Read the model definition and answer for the solid it produces. Units are mm, in the model's axes. Face numbers are marked on the shaded views. A direction names the side the tool comes from. Round coordinates to 2 decimals unless told otherwise and drop trailing zeros. Write each loop counter-clockwise with the first axis right and the second up, starting at its lowest first coordinate (ties: lowest second). Pieces come first, ordered by that corner, then holes. Notation, with made-up numbers: (17, -10) - (49, -10) arc R22 cw to (49, 18) - close; hole circle Ø7 at (70.5, 37.5). An arc over 180 degrees is marked (long way). Answer as CSV lines item,"result". Start each with the question number.
1) Find section B-B on x = -5.5. Determine the outline of the cut face in (y, z).
2) Consider line 1 along Y through (x, z) = (-105, 4.3); line 2 along Y through (x, z) = (-10, -4.5); line 3 along Y through (x, z) = (-31, 0.25). Determine where each line is inside the solid, lowest interval first.
3) For a pull along Y with two mould halves and no side action, classify the marked faces 4, 5, 6 and 7 as +Y half, -Y half, draft (parallel to the pull), parting line (faces both ways), or undercut.
4) Which of the six approach directions +Z, -Z, +X, -X, +Y, -Y give full straight-line access (tool end or side, diameter ignored) to the marked faces 1, 2 and 3?
5) Find section C-C on x = -31. Determine the outline of the cut face in (y, z), then the cut area to 3 significant figures.
6) Find section A-A on x = 10. Determine the outline of the cut face in (y, z).
7) Each of these flat-tipped pins is pushed along its axis until it touches: pin 1 (1.1 mm diameter, centred on y = 9, z = -4, fed in from +X); pin 2 (1.5 mm diameter, centred on y = 1, z = -3, fed in from +X); pin 3 (6 mm diameter, centred on x = 5.5, y = 1, fed in from -Z); pin 4 (3 mm diameter, centred on x = -105, y = -10, fed in from -Z). Where does it stop, or does it pass through?
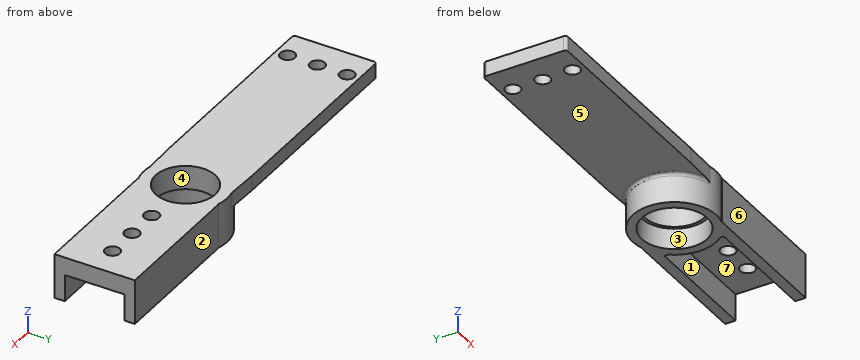
from build123d import *

# Parameters (mm, degrees)
SKETCH_1_W          = 40
SKETCH_1_H          = 20
EXTRUDE_1_DEPTH     = 6
SKETCH_2_R          = 2.5
CUT_EXTRUDE_1_DEPTH = 24.151673806
EXTRUDE_START       = -15
EXTRUDE_2_OUTLINE_R = 11
EXTRUDE_2_DEPTH     = 15
EXTRUDE_START_2     = -8
SKETCH_5_R          = 11
SKETCH_5_R_2        = 10
EXTRUDE_3_DEPTH     = 8
EXTRUDE_START_3     = -5
SKETCH_8_W          = 70
SKETCH_8_H          = 28
EXTRUDE_4_DEPTH     = 5
FILLET_1_R          = 1
FILLET_2_R          = 1
SKETCH_9_R          = 2.5
CUT_EXTRUDE_2_DEPTH = 5


# Read off the part's stored shape, not the designer's step: the extrude step
with BuildPart() as part:
    # Sketch 1 → Extrude 1 (new body)
    with BuildSketch(Plane.XY):
        Rectangle(SKETCH_1_W, SKETCH_1_H)
    extrude(amount=EXTRUDE_1_DEPTH)

    # Sketch 2 → Cut-Extrude 1 (cut, through all)
    with BuildSketch(Plane.XY.offset(6)):
        with Locations((10, 0)):
            Circle(SKETCH_2_R)
        with Locations((-1, 0)):
            Circle(SKETCH_2_R)
        with Locations((-12, 0)):
            Circle(SKETCH_2_R)
    extrude(amount=-CUT_EXTRUDE_1_DEPTH, mode=Mode.SUBTRACT)

    # Extrude 2 outline → Extrude 2 (add)
    with BuildSketch(Plane.XY.offset(6).offset(EXTRUDE_START)):
        with BuildLine():
            Line((20, 10), (20, 13.5))
            Line((20, 13.5), (-26.893967141, 13.5))
            Line((-26.893967141, 13.5), (-26.893967141, 13.384337644))
            ThreePointArc((-26.893967141, 13.384337644), (-45, 0), (-26.893967141, -13.384337644))
            Line((-26.893967141, -13.384337644), (-26.893967141, -13.5))
            Line((-26.893967141, -13.5), (20, -13.5))
            Line((20, -13.5), (20, -10))
            Line((20, -10), (-20, -10))
            Line((-20, -10), (-20, -8.660254038))
            ThreePointArc((-20, -8.660254038), (-17, 0), (-20, 8.660254038))
            Line((-20, 8.660254038), (-20, 10))
            Line((-20, 10), (20, 10))
        make_face()
        with Locations((-31, 0)):
            Circle(EXTRUDE_2_OUTLINE_R, mode=Mode.SUBTRACT)
    extrude(amount=EXTRUDE_2_DEPTH)

    # Sketch 5 → Extrude 3 (add)
    with BuildSketch(Plane.XY.offset(6).offset(EXTRUDE_START_2)):
        with Locations((-31, 0)):
            Circle(SKETCH_5_R)
        with Locations((-31, 0)):
            Circle(SKETCH_5_R_2, mode=Mode.SUBTRACT)
    extrude(amount=EXTRUDE_3_DEPTH)

    # Sketch 8 → Extrude 4 (add)
    with BuildSketch(Plane.XY.offset(6).offset(EXTRUDE_START_3)):
        with Locations((-80, 0)):
            Rectangle(SKETCH_8_W, SKETCH_8_H)
        with BuildLine():
            Line((-45, 5.1e-08), (-45, -14))
            Line((-45, -14), (-33.911999365, -13.693803697))
            ThreePointArc((-33.911999365, -13.693803697), (-41.880440979, -8.809994557), (-45, 5.1e-08))
        make_face()
        with BuildLine():
            Line((-45, 14), (-45, 5.1e-08))
            ThreePointArc((-45, 5.1e-08), (-41.968667344, 8.699904408), (-34.187380521, 13.632336755))
            Line((-34.187380521, 13.632336755), (-45, 14))
        make_face()
    extrude(amount=EXTRUDE_4_DEPTH)

    # Fillet 1
    fillet_1_edges = [part.edges().sort_by_distance(p)[0] for p in [
        (-44.999289152, -0.141078849, 1),
    ]]
    fillet(fillet_1_edges, radius=FILLET_1_R)

    # Fillet 2
    fillet_2_edges = [part.edges().sort_by_distance(p)[0] for p in [
        (-115, -14, 3.5),
        (-115, 14, 3.5),
    ]]
    fillet(fillet_2_edges, radius=FILLET_2_R)

    # Sketch 9 → Cut-Extrude 2 (cut)
    with BuildSketch(Plane.XY.offset(6)):
        with Locations((-105, 0)):
            Circle(SKETCH_9_R)
        with Locations((-105, 10)):
            Circle(SKETCH_9_R)
        with Locations((-105, -10)):
            Circle(SKETCH_9_R)
    extrude(amount=-CUT_EXTRUDE_2_DEPTH, mode=Mode.SUBTRACT)


solid = part.part
Check values:
1,outline,"(-13.5, -9) - (-10, -9) - (-10, 0) - (10, 0) - (10, -9) - (13.5, -9) - (13.5, 6) - (-13.5, 6) - close"
2,line 1,"y = -14 to -12.5, -7.5 to -2.5, 2.5 to 7.5, 12.5 to 14"
2,line 2,"y = -13.5 to -10, 10 to 13.5"
2,line 3,"y = -14 to -10, 10 to 14"
3,face 4,"undercut"
3,face 5,"draft"
3,face 6,"-Y half"
3,face 7,"undercut"
4,face 1,"-Z, +X"
4,face 2,"+Z, -Z, +X, +Y"
4,face 3,"-Z"
5,outline,"(-14, -9) - (-11, -9) - (-11, -2) - (-10, -2) - (-10, 6) - (-14, 6) - close; (10, -2) - (11, -2) - (11, -9) - (14, -9) - (14, 6) - (10, 6) - close"
5,area,"106 mm^2"
6,outline,"(-13.5, -9) - (-10, -9) - (-10, 0) - (-2.5, 0) - (-2.5, 6) - (-13.5, 6) - close; (2.5, 0) - (10, 0) - (10, -9) - (13.5, -9) - (13.5, 6) - (2.5, 6) - close"
7,pin 1,"stops at x = -19.84"
7,pin 2,"stops at x = -17"
7,pin 3,"stops at z = 0"
7,pin 4,"passes through"
